```python
from build123d import *

# Parameters (mm, degrees)
SKETCH_1_W                  = 80
SKETCH_1_H                  = 9.75
HOLE_WIZARD_1_6_1_6_1_D     = 1.6
HOLE_WIZARD_1_6_1_6_1_DEPTH = 15.2
HOLE_WIZARD_1_6_1_6_1_TIP   = 0.480688495
HOLE_WIZARD_1_6_1_6_2_D     = 1.6
HOLE_WIZARD_1_6_1_6_2_DEPTH = 15.2
HOLE_WIZARD_1_6_1_6_2_TIP   = 0.480688495


with BuildPart() as part:
    # 스케치1 → 회전1 (revolve)
    with BuildSketch(Plane(origin=(0, 0, 0), x_dir=(-1, 0, 0), z_dir=(0, 0, -1))):
        with Locations((-40, 4.875)):
            Rectangle(SKETCH_1_W, SKETCH_1_H)
    revolve(axis=Axis((80, 0, 0), (-1, 0, 0)))

    # Ø1.6 (1.6) 지름 구멍1
    with Locations(Plane.ZY):
        with Locations((0, 8), (-5.656854249, 5.656854249), (-8, 0), (-5.656854249, -5.656854249), (0, -8), (5.656854249, -5.656854249), (8, 0), (5.656854249, 5.656854249)):
            Hole(HOLE_WIZARD_1_6_1_6_1_D / 2, depth=HOLE_WIZARD_1_6_1_6_1_DEPTH)
            with Locations((0, 0, -(HOLE_WIZARD_1_6_1_6_1_DEPTH + HOLE_WIZARD_1_6_1_6_1_TIP / 2))):  # 118° drill point
                Cone(0, HOLE_WIZARD_1_6_1_6_1_D / 2, HOLE_WIZARD_1_6_1_6_1_TIP, mode=Mode.SUBTRACT)

    # Ø1.6 (1.6) 지름 구멍2
    with Locations(Plane(origin=(80, 0, 0), x_dir=(0, 0, -1), z_dir=(1, 0, 0))):
        with Locations((0, 8), (5.656854249, 5.656854249), (8, 0), (5.656854249, -5.656854249), (0, -8), (-5.656854249, -5.656854249), (-8, 0), (-5.656854249, 5.656854249)):
            Hole(HOLE_WIZARD_1_6_1_6_2_D / 2, depth=HOLE_WIZARD_1_6_1_6_2_DEPTH)
            with Locations((0, 0, -(HOLE_WIZARD_1_6_1_6_2_DEPTH + HOLE_WIZARD_1_6_1_6_2_TIP / 2))):  # 118° drill point
                Cone(0, HOLE_WIZARD_1_6_1_6_2_D / 2, HOLE_WIZARD_1_6_1_6_2_TIP, mode=Mode.SUBTRACT)


solid = part.part
```
The model under review builds one solid part; all positions refer to its coordinate system, in mm. A direction names the side the tool comes from. Coordinates: 2 decimals unless noted, no trailing zeros. Order: outer loops, then holes, each group sorted by start corner. A loop starts at its lowest first (then second) coordinate and runs counter-clockwise, first axis right, second up. Notation, with made-up numbers: (-25.5, 45) -> (-4.5, 45) arc R30 ccw to (-4.5, 84) -> close; hole circle Ø4 at (81, 38.5). An arc over 180 degrees is marked (long way). Answer in a Markdown table with one row per item. Add a question column.
Item 1: We need section D-D on y = -2.25. Write out the cut boundary in (x, z), plus the area to 3 significant figures.
Item 2: We need section B-B on x = 24.5. Write out the cut boundary in (y, z).
Item 3: We need section C-C on z = -2.5. Write out the cut boundary in (x, y).
Item 4: Clearance check with flat-ended pins moving along their axes: pin 1 (1 mm diameter, centred on x = 64, y = -7.5, fed in from +Z); pin 2 (1 mm diameter, centred on y = 8, z = 0, fed in from -X); pin 3 (1.3 mm diameter, centred on y = 5.66, z = 5.66, fed in from +X); pin 4 (4 mm diameter, centred on x = 62.5, z = -0.5, fed in from -Y). State where each tip first meets the part, or that it passes through.
Item 5: Machinability: for faces 3 (the cylindrical face through (7.706, 8.793, 0.104)), 4 (the cylindrical face through (72.294, 5.35, 6.396)), which of the approach directions +Z, -Z, +X, -X, +Y, -Y give a long, thin tool a straight path to every point of the face, cutting with its end or side? Answer none if there is none.
Item 6: To check wall thickness, follow probe 1 along Y at (x, z) = (10.5, 0); probe 2 along Z at (x, y) = (10, -5.25). State the ranges of each line that lie inside material, in increasing order.
Item 7: Mouldability with a two-part tool opening along Y and no side actions: class faces 1 (the cylindrical face through (7.706, -7.207, 0.104)), 2 (the flat face through (80, 0, 0)) as +Y half, -Y half, draft (parallel to the pull), parting line (faces both ways), or undercut.
Item 8: We need section A-A on x = 10.5. Give the number of separate pieces and of enclosed holes in the cut face, plus the area to 3 significant figures.
Final values:
| question | item | result |
|---|---|---|
| 1 | outline | (0, -9.49) -> (80, -9.49) -> (80, 9.49) -> (0, 9.49) -> close |
| 1 | area | 1,520 mm2 |
| 2 | outline | circle Ø19.5 at (0, 0) |
| 3 | outline | (0, -9.42) -> (80, -9.42) -> (80, 9.42) -> (0, 9.42) -> close |
| 4 | pin 1 | stops at z = 6.79 |
| 4 | pin 2 | stops at x = 15.38 |
| 4 | pin 3 | stops at x = 64.71 |
| 4 | pin 4 | stops at y = -9.75 |
| 5 | face 3 | -X |
| 5 | face 4 | +X |
| 6 | probe 1 | y = -9.75 to -8.8, -7.2 to 7.2, 8.8 to 9.75 |
| 6 | probe 2 | z = -8.22 to -6.35, -4.97 to 4.97, 6.35 to 8.22 |
| 7 | face 1 | undercut |
| 7 | face 2 | draft |
| 8 | separate pieces | 1 |
| 8 | enclosed holes | 8 |
| 8 | area | 283 mm2 |
